```python
from build123d import *

# Parameters (mm, degrees)
SKETCH3_W           = 65
SKETCH3_H           = 60
BOSS_EXTRUDE3_DEPTH = 5
SKETCH5_W           = 43
SKETCH5_H           = 35
CUT_EXTRUDE2_DEPTH  = 10
CUT_EXTRUDE1_REACH  = 57.982
SKETCH4_R           = 1.3
SKETCH9_R           = 2.65
SKETCH9_R_2         = 1.05
BOSS_EXTRUDE5_DEPTH = 6
SKETCH11_W          = 65
SKETCH11_H          = 5
BOSS_EXTRUDE7_DEPTH = 46


with BuildPart() as part:
    # Sketch3 → Boss-Extrude3 (new body)
    with BuildSketch(Plane(origin=(0, 0, 0), x_dir=(1, 0, 0), z_dir=(0, 1, 0))):
        with Locations((-14.5, 0)):
            Rectangle(SKETCH3_W, SKETCH3_H)
    extrude(amount=BOSS_EXTRUDE3_DEPTH)

    # Sketch5 → Cut-Extrude2 (cut)
    with BuildSketch(Plane.XZ):
        with Locations((-14.5, 0)):
            Rectangle(SKETCH5_W, SKETCH5_H)
    extrude(amount=-CUT_EXTRUDE2_DEPTH, mode=Mode.SUBTRACT)

    # Sketch4 → Cut-Extrude1 (cut, up to next)
    with BuildSketch(Plane(origin=(0, 5, 0), x_dir=(1, 0, 0), z_dir=(0, 1, 0)), mode=Mode.PRIVATE) as cut_extrude1_sk1:
        with Locations(Location((-33.5, 20, 0), (0, 0, 270))):
            Circle(SKETCH4_R)
    cut_extrude1_tool1 = extrude(cut_extrude1_sk1.sketch, amount=-CUT_EXTRUDE1_REACH, mode=Mode.PRIVATE) & part.part
    # Sketch4 → Cut-Extrude1 (cut, up to next)
    with BuildSketch(Plane(origin=(0, 5, 0), x_dir=(1, 0, 0), z_dir=(0, 1, 0)), mode=Mode.PRIVATE) as cut_extrude1_sk2:
        with Locations(Location((4.5, 20, 0), (0, 0, 270))):
            Circle(SKETCH4_R)
    cut_extrude1_tool2 = extrude(cut_extrude1_sk2.sketch, amount=-CUT_EXTRUDE1_REACH, mode=Mode.PRIVATE) & part.part
    # Sketch4 → Cut-Extrude1 (cut, up to next)
    with BuildSketch(Plane(origin=(0, 5, 0), x_dir=(1, 0, 0), z_dir=(0, 1, 0)), mode=Mode.PRIVATE) as cut_extrude1_sk3:
        with Locations(Location((4.5, -20, 0), (0, 0, 270))):
            Circle(SKETCH4_R)
    cut_extrude1_tool3 = extrude(cut_extrude1_sk3.sketch, amount=-CUT_EXTRUDE1_REACH, mode=Mode.PRIVATE) & part.part
    # Sketch4 → Cut-Extrude1 (cut, up to next)
    with BuildSketch(Plane(origin=(0, 5, 0), x_dir=(1, 0, 0), z_dir=(0, 1, 0)), mode=Mode.PRIVATE) as cut_extrude1_sk4:
        with Locations(Location((-33.5, -20, 0), (0, 0, 270))):
            Circle(SKETCH4_R)
    cut_extrude1_tool4 = extrude(cut_extrude1_sk4.sketch, amount=-CUT_EXTRUDE1_REACH, mode=Mode.PRIVATE) & part.part
    add(cut_extrude1_tool1.solids().sort_by_distance((-33.5, 5, -20))[0], mode=Mode.SUBTRACT)
    add(cut_extrude1_tool2.solids().sort_by_distance((4.5, 5, -20))[0], mode=Mode.SUBTRACT)
    add(cut_extrude1_tool3.solids().sort_by_distance((4.5, 5, 20))[0], mode=Mode.SUBTRACT)
    add(cut_extrude1_tool4.solids().sort_by_distance((-33.5, 5, 20))[0], mode=Mode.SUBTRACT)

    # Sketch9 → Boss-Extrude5 (add)
    # profile 1 of 4: a face of its own
    with BuildSketch(Plane.XZ):
        with Locations(Location((-33.5, 20, 0), (0, 0, 250.629961754))):
            Circle(SKETCH9_R)
        with Locations(Location((-33.5, 20, 0), (0, 0, 270))):
            Circle(SKETCH9_R_2, mode=Mode.SUBTRACT)
    # profile 2 of 4: a face of its own
    with BuildSketch(Plane.XZ):
        with Locations(Location((-33.5, -20, 0), (0, 0, 109.370038246))):
            Circle(SKETCH9_R)
        with Locations(Location((-33.5, -20, 0), (0, 0, 270))):
            Circle(SKETCH9_R_2, mode=Mode.SUBTRACT)
    # profile 3 of 4: a face of its own
    with BuildSketch(Plane.XZ):
        with Locations(Location((4.5, 20, 0), (0, 0, 289.370038246))):
            Circle(SKETCH9_R)
        with Locations(Location((4.5, 20, 0), (0, 0, 270))):
            Circle(SKETCH9_R_2, mode=Mode.SUBTRACT)
    # profile 4 of 4: a face of its own
    with BuildSketch(Plane.XZ):
        with Locations(Location((4.5, -20, 0), (0, 0, 109.370038246))):
            Circle(SKETCH9_R)
        with Locations(Location((4.5, -20, 0), (0, 0, 270))):
            Circle(SKETCH9_R_2, mode=Mode.SUBTRACT)
    extrude(amount=BOSS_EXTRUDE5_DEPTH)

    # Sketch11 → Boss-Extrude7 (add)
    with BuildSketch(Plane.XY.offset(30)):
        with Locations((-14.5, 2.5)):
            Rectangle(SKETCH11_W, SKETCH11_H)
    extrude(amount=BOSS_EXTRUDE7_DEPTH)


solid = part.part
```
Verification items for the finished model (mm, model axes). A direction names the side the tool comes from. Round coordinates to 2 decimals unless told otherwise and drop trailing zeros. Order: outer loops, then holes, each group sorted by start corner. A loop starts at its lowest first (then second) coordinate and runs counter-clockwise, first axis right, second up.
1) Cross-section at D-D, the plane z = -2.5. Record the cut outline in (x, y).
Geometry says:
outline: (-47, 0) - (-36, 0) - (-36, 5) - (-47, 5) - close; (7, 0) - (18, 0) - (18, 5) - (7, 5) - close
2) Tool access check on faces 4 (the flat face through (-36, 2, 0)), 5 (the flat face through (-47, 2, 22)), 6 (the cylindrical face through (3.71, 2.54, 18.97)), 7 (the flat face through (-15, 5, 34)), 8 (the cylindrical face through (-31.864, -2.958, 17.915)). Record the directions out of +Z, -Z, +X, -X, +Y, -Y that give a thin tool (end or side, any length) a straight path to the whole face; none if there is none.
Geometry says:
face 4: +Y, -Y
face 5: +Z, -Z, -X, +Y, -Y
face 6: +Y
face 7: +Z, -Z, +X, -X, +Y
face 8: -Y
3) Cross-section at A-A, the plane z = 20. Record the cut outline in (x, y).
Geometry says:
outline: (-47, 0) - (-36.15, 0) - (-36.15, -6) - (-34.55, -6) - (-34.55, 0) - (-34.8, 0) - (-34.8, 5) - (-47, 5) - close; (-32.45, -6) - (-30.85, -6) - (-30.85, 0) - (1.85, 0) - (1.85, -6) - (3.45, -6) - (3.45, 0) - (3.2, 0) - (3.2, 5) - (-32.2, 5) - (-32.2, 0) - (-32.45, 0) - close; (5.55, -6) - (7.15, -6) - (7.15, 0) - (18, 0) - (18, 5) - (5.8, 5) - (5.8, 0) - (5.55, 0) - close
4) Draft check along Z on faces 1 (the cylindrical face through (5.268, -2.958, -22.536)), 2 (the flat face through (6, -6, -20)), 3 (the flat face through (-15, 2, -30)). Enter one of: +Z half, -Z half, draft (parallel to the pull), parting line (faces both ways), or undercut.
Geometry says:
face 1: undercut
face 2: draft
face 3: -Z half
5) Cross-section at C-C, the plane y = -4. Record the cut outline in (x, z).
Geometry says:
outline: circle Ø5.3 at (-33.5, -20); circle Ø5.3 at (-33.5, 20); circle Ø5.3 at (4.5, -20); circle Ø5.3 at (4.5, 20); hole circle Ø2.1 at (-33.5, -20); hole circle Ø2.1 at (-33.5, 20); hole circle Ø2.1 at (4.5, -20); hole circle Ø2.1 at (4.5, 20)
6) Material ranges on line 1 (X direction, y = 2.85, z = -20); line 2 (X direction, y = -2.25, z = 20); line 3 (X direction, y = 0.25, z = 12), recorded low to high.
Geometry says:
line 1: x = -47 to -34.8, -32.2 to 3.2, 5.8 to 18
line 2: x = -36.15 to -34.55, -32.45 to -30.85, 1.85 to 3.45, 5.55 to 7.15
line 3: x = -47 to -36, 7 to 18
7) Depth check by flat-ended pin: pin 1 (1.6 mm diameter, centred on x = 4.5, z = -20, fed in from -Y); pin 2 (1.3 mm diameter, centred on x = -34, z = -20, fed in from +Y). Enter the tip coordinate at first touch or a pass-through.
Geometry says:
pin 1: passes through
pin 2: stops at y = 0
8) Cross-section at B-B, the plane x = -9.5. Record the cut outline in (y, z), plus the area to 3 significant figures.
Geometry says:
outline: (0, -30) - (5, -30) - (5, -17.5) - (0, -17.5) - close; (0, 17.5) - (5, 17.5) - (5, 76) - (0, 76) - close
area: 355 mm2
